Here's how the part is built. I have some questions about the finished solid (model axes, mm). A direction names the side the tool comes from. Coordinates: 2 decimals unless noted, no trailing zeros. Order: outer loops, then holes, each group sorted by start corner. A loop starts at its lowest first (then second) coordinate and runs counter-clockwise, first axis right, second up. Notation, with made-up numbers: (21, -1) - (25, -1) arc R12 ccw to (25, 16) - close; hole circle Ø10 at (-2, 26.5). An arc over 180 degrees is marked (long way). Answer as CSV lines item,"result". Start each with the question number.
Item 1: I need wall thicknesses on line 1 (Y direction, x = 0, z = 3.8); line 2 (Y direction, x = -1, z = 3.7); line 3 (Y direction, x = 0, z = 1.05). Which ranges of each line are inside material? Lowest first, please.
Item 2: Imagine slicing it at A-A on x = 0. List the corners of the cut face in (y, z) for me, and give its area (3 significant figures).
Item 3: I'm going to push a flat-ended pin straight in: pin 1 (1.5 mm diameter, centred on y = -2.5, z = 3.5, fed in from -X). Where does the tip first touch, or does it pass through?
Item 4: Imagine slicing it at C-C on z = 0.7. List the corners of the cut face in (x, y) for me.
Item 5: On a 3-axis mill with a long thin cutter (end or side, diameter ignored), from which of +Z, -Z, +X, -X, +Y, -Y can I reach the whole of each face in a straight line? I mean faces 1 (the face through (1, -3, 0.5)), 2 (the face through (-2, 2, 0)), 3 (the face through (-0.59, 4.46, 3.75)). Say none if no direction works.
Item 6: Imagine slicing it at D-D on x = -4. List the corners of the cut face in (y, z) for me.
Item 7: We'd pull the mould along Y, two halves only. Please class faces 4 (the face through (-2, 2, 4)), 5 (the face through (-1.08, -4.88, 1.97)), 6 (the face through (1, -3, 3.5)): pulls with the +Y half, pulls with the -Y half, needs draft (parallel to the pull), parting line crosses it, or undercut.
from build123d import *

# Parameters (mm, degrees)
SKETCH_2_R          = 5
SKETCH_2_R_2        = 2.5
EXTRUDE_1_DEPTH     = 4
SKETCH_3_R          = 4.5
SKETCH_3_R_2        = 3
CUT_EXTRUDE_1_DEPTH = 0.5
CUT_EXTRUDE_START   = -4
SKETCH_3_2_R        = 4.5
SKETCH_3_2_R_2      = 3
CUT_EXTRUDE_2_DEPTH = 0.5


with BuildPart() as part:
    # 草图2 → 凸台-拉伸1 (new body)
    with BuildSketch(Plane.XY):
        Circle(SKETCH_2_R)
        Circle(SKETCH_2_R_2, mode=Mode.SUBTRACT)
    extrude(amount=EXTRUDE_1_DEPTH)

    # 草图3 → 切除-拉伸1 (cut)
    with BuildSketch(Plane.XY.offset(4)):
        Circle(SKETCH_3_R)
        Circle(SKETCH_3_R_2, mode=Mode.SUBTRACT)
    extrude(amount=-CUT_EXTRUDE_1_DEPTH, mode=Mode.SUBTRACT)

    # 草图3<2> → 切除-拉伸2 (cut)
    with BuildSketch(Plane.XY.offset(4).offset(CUT_EXTRUDE_START)):
        Circle(SKETCH_3_2_R)
        Circle(SKETCH_3_2_R_2, mode=Mode.SUBTRACT)
    extrude(amount=CUT_EXTRUDE_2_DEPTH, mode=Mode.SUBTRACT)


solid = part.part
Responses:
1,line 1,"y = -5 to -4.5, -3 to -2.5, 2.5 to 3, 4.5 to 5"
1,line 2,"y = -4.9 to -4.39, -2.83 to -2.29, 2.29 to 2.83, 4.39 to 4.9"
1,line 3,"y = -5 to -2.5, 2.5 to 5"
2,outline,"(-5, 0) - (-4.5, 0) - (-4.5, 0.5) - (-3, 0.5) - (-3, 0) - (-2.5, 0) - (-2.5, 4) - (-3, 4) - (-3, 3.5) - (-4.5, 3.5) - (-4.5, 4) - (-5, 4) - close; (2.5, 0) - (3, 0) - (3, 0.5) - (4.5, 0.5) - (4.5, 0) - (5, 0) - (5, 4) - (4.5, 4) - (4.5, 3.5) - (3, 3.5) - (3, 4) - (2.5, 4) - close"
2,area,"17.0 mm^2"
3,pin 1,"stops at x = -4.68"
4,outline,"circle Ø10 at (0, 0); hole circle Ø5 at (0, 0)"
5,face 1,"-Z"
5,face 2,"-Z, +X, -X, +Y, -Y"
5,face 3,"+Z"
6,outline,"(-3, 0) - (-2.06, 0) - (-2.06, 0.5) - (2.06, 0.5) - (2.06, 0) - (3, 0) - (3, 4) - (2.06, 4) - (2.06, 3.5) - (-2.06, 3.5) - (-2.06, 4) - (-3, 4) - close"
7,face 4,"needs draft"
7,face 5,"parting line crosses it"
7,face 6,"undercut"
